The model under review builds one solid part; all positions refer to its coordinate system, in mm. Face numbers are marked on the shaded views. A direction names the side the tool comes from. Round coordinates to 2 decimals unless told otherwise and drop trailing zeros. Loops run counter-clockwise (first coordinate to the right, second up) from the corner with the lowest first, then second, coordinate; pieces in that order, holes last. Notation, with made-up numbers: M 49.25,42 L 73.25,42 A24 cw 73.25,78 Z; hole C -36,-14.5 d3. An arc over 180 degrees is marked long. Answer in a Markdown table with one row per item. Add a question column.
from build123d import *

# Parameters (mm, degrees)
IZIM1_R                     = 10
IZIM1_R_2                   = 1.5
Y_KSEKLIK_EKSTR_ZYON1_DEPTH = 2.5
IZIM2_R                     = 4.5
IZIM2_R_2                   = 2.95
Y_KSEKLIK_EKSTR_ZYON2_DEPTH = 2
IZIM3_R                     = 1.6
KES_EKSTR_ZYON1_DEPTH       = 3.5
IZIM4_R                     = 2.95
IZIM4_R_2                   = 1.6
KES_EKSTR_ZYON2_DEPTH       = 2


with BuildPart() as part:
    # Çizim1 → Yükseklik-Ekstrüzyon1 (new body)
    with BuildSketch(Plane(origin=(0, 0, 0), x_dir=(1, 0, 0), z_dir=(0, 1, 0))):
        Circle(IZIM1_R)
        with Locations((0, 7)):
            Circle(IZIM1_R_2, mode=Mode.SUBTRACT)
        with Locations((7, 0)):
            Circle(IZIM1_R_2, mode=Mode.SUBTRACT)
        with Locations((0, -7)):
            Circle(IZIM1_R_2, mode=Mode.SUBTRACT)
        with Locations((-7, 0)):
            Circle(IZIM1_R_2, mode=Mode.SUBTRACT)
    extrude(amount=Y_KSEKLIK_EKSTR_ZYON1_DEPTH)

    # Çizim2 → Yükseklik-Ekstrüzyon2 (add)
    with BuildSketch(Plane(origin=(0, 2.5, 0), x_dir=(1, 0, 0), z_dir=(0, 1, 0))):
        Circle(IZIM2_R)
        Circle(IZIM2_R_2, mode=Mode.SUBTRACT)
    extrude(amount=Y_KSEKLIK_EKSTR_ZYON2_DEPTH)

    # Çizim3 → Kes-Ekstrüzyon1 (cut, through all)
    with BuildSketch(Plane(origin=(0, 2.5, 0), x_dir=(1, 0, 0), z_dir=(0, 1, 0))):
        Circle(IZIM3_R)
    extrude(amount=-KES_EKSTR_ZYON1_DEPTH, mode=Mode.SUBTRACT)

    # Çizim4 → Kes-Ekstrüzyon2 (cut)
    with BuildSketch(Plane(origin=(0, 2.5, 0), x_dir=(1, 0, 0), z_dir=(0, 1, 0))):
        Circle(IZIM4_R)
        Circle(IZIM4_R_2, mode=Mode.SUBTRACT)
    extrude(amount=-KES_EKSTR_ZYON2_DEPTH, mode=Mode.SUBTRACT)


solid = part.part
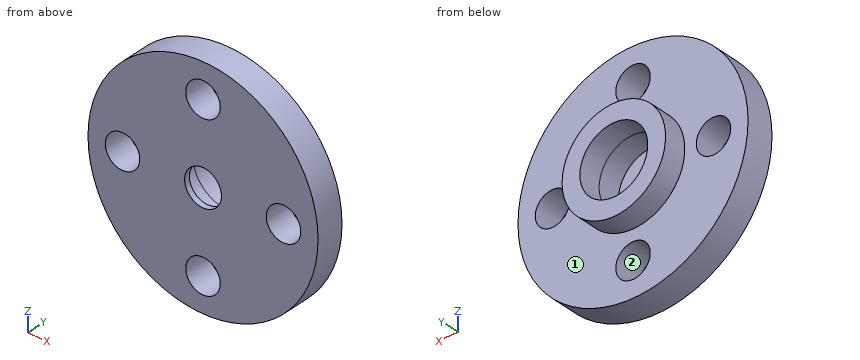
1. Take a section at B-B, the plane x = 0. State the section outline as (y, z) points, and give its area (3 significant figures).
2. To check wall thickness, follow probe 1 along Z at (x, y) = (0, 0.3); probe 2 along X at (y, z) = (1.3, 0). State the ranges of each line that lie inside material, in increasing order.
3. For pin 1 Ø4 at (x, z) = (0, 0) entering from +Y; pin 2 Ø1.5 at (y, z) = (3, -7) entering from +X; pin 3 Ø1.5 at (y, z) = (3, 2.5) entering from -X, all flat-tipped, find the tip position at first contact; note any pin that passes through.
4. Take a section at C-C, the plane x = 7. State the section outline as (y, z) points, and give its area (3 significant figures).
5. Machinability: for the marked faces 1 and 2, which of the approach directions +Z, -Z, +X, -X, +Y, -Y give a long, thin tool a straight path to every point of the face, cutting with its end or side? Answer none if there is none.
6. Take a section at A-A, the plane z = 0. State the section outline as (x, y) points.
7. Take a section at D-D, the plane y = 1.6. State the section outline as (x, z) points.
Check sheet entries:
| question | item | result |
|---|---|---|
| 1 | outline | M 0,-10 L 2.5,-10 L 2.5,-8.5 L 0,-8.5 Z; M 0,-5.5 L 2.5,-5.5 L 2.5,-4.5 L 4.5,-4.5 L 4.5,-2.95 L 0.5,-2.95 L 0.5,-1.6 L 0,-1.6 Z; M 0,1.6 L 0.5,1.6 L 0.5,2.95 L 4.5,2.95 L 4.5,4.5 L 2.5,4.5 L 2.5,5.5 L 0,5.5 Z; M 0,8.5 L 2.5,8.5 L 2.5,10 L 0,10 Z |
| 1 | area | 27.8 mm^2 |
| 2 | probe 1 | z = -10 to -8.5, -5.5 to -1.6, 1.6 to 5.5, 8.5 to 10 |
| 2 | probe 2 | x = -10 to -8.5, -5.5 to -2.95, 2.95 to 5.5, 8.5 to 10 |
| 3 | pin 1 | stops at y = 0.5 |
| 3 | pin 2 | stops at x = 7.65 |
| 3 | pin 3 | stops at x = -9.81 |
| 4 | outline | M 0,-7.14 L 2.5,-7.14 L 2.5,-1.5 L 0,-1.5 Z; M 0,1.5 L 2.5,1.5 L 2.5,7.14 L 0,7.14 Z |
| 4 | area | 28.2 mm^2 |
| 5 | face 1 | +Y |
| 5 | face 2 | +Y, -Y |
| 6 | outline | M -10,0 L -8.5,0 L -8.5,2.5 L -10,2.5 Z; M -5.5,0 L -1.6,0 L -1.6,0.5 L -2.95,0.5 L -2.95,4.5 L -4.5,4.5 L -4.5,2.5 L -5.5,2.5 Z; M 1.6,0 L 5.5,0 L 5.5,2.5 L 4.5,2.5 L 4.5,4.5 L 2.95,4.5 L 2.95,0.5 L 1.6,0.5 Z; M 8.5,0 L 10,0 L 10,2.5 L 8.5,2.5 Z |
| 7 | outline | C 0,0 d20; hole C -7,0 d3; hole C 0,0 d5.9; hole C 0,-7 d3; hole C 0,7 d3; hole C 7,0 d3 |
